Work out the finished part from the listing and answer in its coordinate system (mm). Round coordinates to 2 decimals unless told otherwise and drop trailing zeros. Order: outer loops, then holes, each group sorted by start corner. A loop starts at its lowest first (then second) coordinate and runs counter-clockwise, first axis right, second up. Notation, with made-up numbers: M 59,39.25 L 105,39.25 A31 ccw 105,74.25 Z; hole C -10.75,86 d10. An arc over 180 degrees is marked long. Answer as a JSON object with one key per item and string values. Group by question number.
Autodesk Inventor part; units mm, degrees
ref_plane "Work Plane1" through (16.5341, 952.9567, 0) normal (0, 0, 1) x (-1, 0, 0)
ref_plane "YZ Plane" through (0, 0, 0) normal (1, 0, 0) x (0, 1, 0)
ref_plane "XZ Plane" through (0, 0, 0) normal (0, 1, 0) x (-1, 0, 0)
ref_plane "Work Plane1" through (16.5341, 952.9567, 0) normal (0, 0, 1) x (-1, 0, 0)
sketch "Sketch4" plane through (16.5341, 952.9567, 3) normal (0, 0, 1) x (1, 0, 0)
  line L0 (-26.5, -89.1167) -> (-26.5, 59.6119)
  line L1 (26.5, 59.6119) -> (26.5, -89.1167)
  line L2 (-26.5, 59.6119) -> (26.5, 59.6119)
  line L3 (-25, 59.6119) -> (-25, -89.1167)
  line L4 (26.5, 59.6119) -> (-26.5, 59.6119)
  line L5 (25, 59.6119) -> (25, -89.1167)
  line L6 (-26.5, -89.1167) -> (-25, -89.1167)
  line L7 (58, -89.1167) -> (26.5, -89.1167)
  line L8 (26.5, -89.1167) -> (25, -89.1167)
  point P0 (-16.5341, -952.9567)
  dimension "d15" = 1.5
  dimension "d16" = 1.5
sketch "Sketch1" plane through (16.5341, 952.9567, 0) normal (0, 0, 1) x (-1, 0, 0)
  line L0 (60, 40.2719) -> (60, 137.1193)
  ellipse E0 centre (56, 137.1193) end of major axis (56, 141.9614) minor radius 4 (60, 137.1193) -> (56, 141.9614) ccw
  line L1 (56, 141.9614) -> (24.75, 141.9614)
  line L2 (24.75, 141.9614) -> (24.75, 144.3824)
  line L3 (24.75, 144.3824) -> (24.75, 146.8034)
  line L4 (24.75, 146.8034) -> (56, 146.8034)
  ellipse E1 centre (56, 137.1193) end of major axis (56, 146.8034) minor radius 8 (64, 137.1193) -> (56, 146.8034) ccw
  line L5 (64, 137.1193) -> (64, 40.2719)
  ellipse E2 centre (56, 40.2719) end of major axis (56, 30.5879) minor radius 8 (63.7591, 37.9134) -> (64, 40.2719) ccw
  line L6 (63.7591, 37.9134) -> (43.4204, -60.1335)
  ellipse E3 centre (35.6613, -57.775) end of major axis (35.6613, -67.459) minor radius 8 (42.7123, -62.3499) -> (43.4204, -60.1335) ccw
  line L7 (42.7123, -62.3499) -> (7.051, -142.8866)
  ellipse E4 centre (0, -138.3116) end of major axis (0, -147.9957) minor radius 8 (-7.051, -142.8866) -> (7.051, -142.8866) ccw
  line L8 (-7.051, -142.8866) -> (-42.7123, -62.3499)
  ellipse E5 centre (-35.6613, -57.775) end of major axis (-35.6613, -67.459) minor radius 8 (-43.4204, -60.1335) -> (-42.7123, -62.3499) ccw
  line L9 (-43.4204, -60.1335) -> (-63.7591, 37.9134)
  ellipse E6 centre (-56, 40.2719) end of major axis (-56, 30.5879) minor radius 8 (-64, 40.2719) -> (-63.7591, 37.9134) ccw
  line L10 (-64, 40.2719) -> (-64, 137.1193)
  ellipse E7 centre (-56, 137.1193) end of major axis (-56, 146.8034) minor radius 8 (-56, 146.8034) -> (-64, 137.1193) ccw
  line L11 (-56, 146.8034) -> (-24.75, 146.8034)
  line L12 (-24.75, 146.8034) -> (-24.75, 144.3824)
  line L13 (-24.75, 144.3824) -> (-24.75, 141.9614)
  line L14 (-24.75, 141.9614) -> (-56, 141.9614)
  ellipse E8 centre (-56, 137.1193) end of major axis (-56, 141.9614) minor radius 4 (-56, 141.9614) -> (-60, 137.1193) ccw
  line L15 (-60, 137.1193) -> (-60, 40.2719)
  ellipse E9 centre (-56, 40.2719) end of major axis (-56, 35.4299) minor radius 4 (-60, 40.2719) -> (-59.8796, 39.0927) ccw
  line L16 (-59.8796, 39.0927) -> (-39.5409, -58.9542)
  ellipse E10 centre (-35.6613, -57.775) end of major axis (-35.6613, -62.617) minor radius 4 (-39.5409, -58.9542) -> (-39.1868, -60.0624) ccw
  line L17 (-39.1868, -60.0624) -> (-3.5255, -140.5991)
  ellipse E11 centre (0, -138.3116) end of major axis (0, -143.1536) minor radius 4 (-3.5255, -140.5991) -> (3.5255, -140.5991) ccw
  line L18 (3.5255, -140.5991) -> (39.1868, -60.0624)
  ellipse E12 centre (35.6613, -57.775) end of major axis (35.6613, -62.617) minor radius 4 (39.1868, -60.0624) -> (39.5409, -58.9542) ccw
  line L19 (39.5409, -58.9542) -> (59.8796, 39.0927)
  ellipse E13 centre (56, 40.2719) end of major axis (56, 35.4299) minor radius 4 (59.8796, 39.0927) -> (60, 40.2719) ccw
  line L20 (-24.75, 141.9614) -> (24.75, 141.9614)
  line L21 (-60, 91.1167) -> (60, 91.1167)
  line L22 (-24.0389, -94.2722) -> (24.0389, -94.2722)
  line L23 (-24.5, 91.1167) -> (-24.5, -57.6119)
  line L24 (-24.5, -57.6119) -> (24.5, -57.6119)
  line L25 (24.5, -57.6119) -> (24.5, 91.1167)
  point P0 (16.5341, 952.9567)
  dimension "d0" = 49
  dimension "d1" = 120
  dimension "d2" = 35.5
  dimension "d3" = 88.0788
  dimension "d4" = 44.0394
  dimension "d5" = 101.6894
  dimension "d6" = 50.8447
  dimension "d7" = 15
extrude "Plate1" add sketch "Sketch1" along normal blind 3 contours E13 L19 E12 L18 L22 L17 E10 L16 E9 L15 L21 L23 L24 L25 L0
sketch "Sketch2" plane through (16.5341, 952.9567, 0) normal (0, 0, -1) x (-1, 0, 0)
  line L0 (60, -40.2719) -> (60, -91.1167)
  ellipse E0 centre (56, -40.2719) end of major axis (56, -35.4299) minor radius 4 (60, -40.2719) -> (59.8796, -39.0927) ccw
  line L1 (39.5409, 58.9542) -> (59.8796, -39.0927)
  ellipse E1 centre (35.6613, 57.775) end of major axis (35.6613, 62.617) minor radius 4 (39.5409, 58.9542) -> (39.1868, 60.0624) ccw
  line L2 (24.0389, 94.2722) -> (39.1868, 60.0624)
  line L3 (-24.0389, 94.2722) -> (24.0389, 94.2722)
  line L4 (-39.1868, 60.0624) -> (-24.0389, 94.2722)
  ellipse E2 centre (-35.6613, 57.775) end of major axis (-35.6613, 62.617) minor radius 4 (-39.1868, 60.0624) -> (-39.5409, 58.9542) ccw
  line L5 (-59.8796, -39.0927) -> (-39.5409, 58.9542)
  ellipse E3 centre (-56, -40.2719) end of major axis (-56, -35.4299) minor radius 4 (-59.8796, -39.0927) -> (-60, -40.2719) ccw
  line L6 (-60, -91.1167) -> (-60, -40.2719)
  line L7 (-24.5, -91.1167) -> (-60, -91.1167)
  line L8 (-24.5, 57.6119) -> (-24.5, -91.1167)
  line L9 (24.5, 57.6119) -> (-24.5, 57.6119)
  line L10 (24.5, -91.1167) -> (24.5, 57.6119)
  line L11 (60, -91.1167) -> (24.5, -91.1167)
  line L12 (-57.9212, -39.4989) -> (-37.5826, 58.548)
  line L13 (-37.3581, 59.2527) -> (-22.7372, 92.2722)
  line L14 (-22.7372, 92.2722) -> (22.7372, 92.2722)
  line L15 (22.7372, 92.2722) -> (37.3581, 59.2527)
  line L16 (37.5826, 58.548) -> (57.9212, -39.4989)
  line L17 (58, -40.2719) -> (58, -89.1167)
  line L18 (58, -89.1167) -> (26.5, -89.1167)
  line L19 (26.5, -89.1167) -> (26.5, 59.6119)
  line L20 (26.5, 59.6119) -> (-26.5, 59.6119)
  line L21 (-26.5, 59.6119) -> (-26.5, -89.1167)
  line L22 (-26.5, -89.1167) -> (-58, -89.1167)
  line L23 (-58, -89.1167) -> (-58, -40.2719)
  spline S0 degree 3 poles (-58, -40.2719) (-58, -40.0125) (-57.9739, -39.753) (-57.9212, -39.4989) knots 0 0 0 0 1 1 1 1
  spline S1 degree 3 poles (-37.5826, 58.548) (-37.5324, 58.7898) (-37.4581, 59.0268) (-37.3581, 59.2527) knots 0 0 0 0 1 1 1 1
  spline S2 degree 3 poles (37.3581, 59.2527) (37.4581, 59.0268) (37.5324, 58.7898) (37.5826, 58.548) knots 0 0 0 0 1 1 1 1
  spline S3 degree 3 poles (57.9212, -39.4989) (57.9739, -39.753) (58, -40.0125) (58, -40.2719) knots 0 0 0 0 1 1 1 1
  point P0 (16.5341, -952.9567)
  dimension "d9" = 2
extrude "Cut1" cut sketch "Sketch2" against normal blind 3
ref_plane "midtplan" through (16.5341, 863.84, 0) normal (1, 0, 0) x (0, 0, -1)
ref_plane "modplan parallel med plade" through (16.5341, 952.9567, 1.5) normal (0, 0, 1) x (1, 0, 0)
sheet face with bend "Face2" sketch "Sketch4" thickness 3 toward (0, 0, -1) bend radius 3
bend "Bend1"
equation "\"d2\" = -0.5 * d0 + 0.5 * d1"
equation "\"d6\" = 0.5 * d5"
equation "\"d10\" = Thickness"
equation "\"d16\" = d15"
equation "\"d8\" = Thickness"
equation "\"d17\" = BendRadius"
equation "\"d18\" = BendReliefWidth"
equation "\"d20\" = MinimumRemnant"
equation "\"d19\" = BendReliefDepth"
equation "\"d21\" = TransitionRadius"
equation "\"Thickness\" = pladetykkelse"
equation "\"BendRadius\" = Thickness"
equation "\"BendReliefWidth\" = Thickness"
equation "\"BendReliefDepth\" = 0.5 * Thickness"
equation "\"CornerReliefSize\" = 4 * Thickness"
equation "\"MinimumRemnant\" = 2 * Thickness"
equation "\"TransitionRadius\" = BendRadius"
equation "\"JacobiRadiusSize\" = BendRadius"
equation "\"GapSize\" = Thickness"
equation "\"pladetykkelse\" = 3"
equation "\"trappevinkel\" = 34.3deg"
equation "\"trappestifter_dia\" = 25"
equation "\"trappestifter_huldia\" = 25.8"
equation "\"trappestifter_skraa_huldia\" = 26.6"
equation "\"trappestifter_laengde\" = 228"
equation "\"perforeringsbredde\" = 6"
equation "\"perforeringshullaengde\" = 62.8"
equation "\"perforeringshullaengde_top\" = 61"
equation "\"perforeringshullaengde_bund\" = 61.6"
equation "\"perforeringsoffset\" = 8"
equation "\"perforeringsoffset_top\" = 8"
equation "\"perforeringsoffset_bund\" = 8"
equation "\"laskehul_dia\" = 13"
equation "\"balusterhul_udvidelse\" = 1"
equation "\"trinbredde\" = 1884"
properties part number "baluster-fod" material "S355MC"
Item 1: Consider L1, parallel to X at y = 877, z = 2; L2, parallel to X at y = 924, z = 2.05; L3, parallel to Y at x = -6, z = 0.6. Determine where each line is inside the solid, lowest interval first.
Item 2: Find section D-D (x = -29.5). Give the vertices of the cut face in (y, z).
Item 3: Find section A-A (y = 922). Give the vertices of the cut face in (x, z), and give its area (3 significant figures).
Item 4: This flat-tipped pin is pushed along its axis until it touches: pin 1 (1.5 mm diameter, centred on x = 7, z = 1.5, fed in from -Y). Where does it stop, or does it pass through?
Item 5: Find section C-C (x = 35). Give the vertices of the cut face in (y, z).
Item 6: Find section B-B (y = 884). Give the vertices of the cut face in (x, z).
Responses:
{
 "1": {"L1": "x = -41.47 to -8.47, 41.53 to 74.53", "L2": "x = -39.2 to -8.47, 41.53 to 72.27", "L3": "y = 1012.57 to 1045.23"},
 "2": {"outline": "M 863.84,0 L 970.76,0 L 970.76,3 L 863.84,3 Z"},
 "3": {"outline": "M -39.62,0 L -8.47,0 L -8.47,3 L -39.62,3 Z; M 41.53,0 L 72.68,0 L 72.68,3 L 41.53,3 Z", "area": "187 mm^2"},
 "4": {"pin 1": "stops at y = 1012.57"},
 "5": {"outline": "M 1012.57,0 L 1045.23,0 L 1045.23,3 L 1012.57,3 Z"},
 "6": {"outline": "M -41.47,0 L -8.47,0 L -8.47,3 L -41.47,3 Z; M 41.53,0 L 74.53,0 L 74.53,3 L 41.53,3 Z"}
}
